Input: part model. Units: mm. Frame: model coordinates. Face numbers are marked on the shaded views. Coordinates: 2 decimals unless noted, no trailing zeros. Loops run counter-clockwise (first coordinate to the right, second up) from the corner with the lowest first, then second, coordinate; pieces in that order, holes last. Notation, with made-up numbers: (56, -23) -> (93, -23) arc R5 cw to (93, -17) -> close; hole circle Ø2 at (-31.75, 76.5). An arc over 180 degrees is marked (long way). Put each result on its own line as item: value. Start each with the question number.
1) Contact query for flat-ended pins moving along their axis: P1, Ø1.8, axis at x = -17.5, z = 3.5, coming from the -Y side; P2, Ø4, axis at x = 48.05, y = 110.5, coming from the -Z side; P3, Ø1.8, axis at y = 118, z = 4.5, coming from the -X side; P4, Ø3, axis at y = 100, z = 2.5, coming from the +X side. Output: stop coordinate, or through.
2) Pull-direction query (X, two-part tool) for the marked faces 1 and 2; classes: pulls with the +X half, pulls with the -X half, needs draft (parallel to the pull), parting line crosses it, or undercut.
3) Cut plane A-A (x = 10.5). Return the cut outline in (y, z), plus the area to 3 significant figures.
4) Cut plane C-C (y = 120.5). Return the cut outline in (x, z), plus the area to 4 significant figures.
5) Cut plane B-B (y = 37). Return the cut outline in (x, z), plus the area to 3 significant figures.
6) Material intervals for L1, parallel to X at y = 150, z = 8.15; L2, parallel to Y at x = -22, z = 4.75; L3, parallel to Y at x = 1.5, z = 7, sorted ascending.
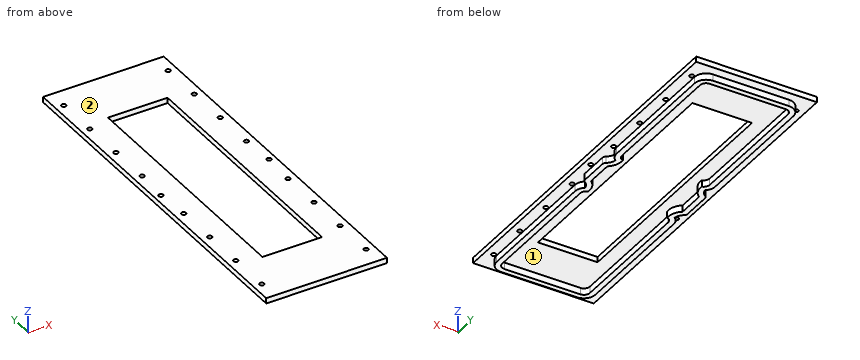
from build123d import *

# Parameters (mm, degrees)
BOSS_EXTRUDE1_DEPTH = 6
BOSS_EXTRUDE2_START = 6
SKETCH1_W           = 111.3
SKETCH1_H           = 338
SKETCH1_R           = 2.1
SKETCH1_W_2         = 54.9
SKETCH1_H_2         = 234
BOSS_EXTRUDE2_DEPTH = 5


with BuildPart() as part:
    # Sketch2 → Boss-Extrude1 (new body)
    with BuildSketch(Plane.XY.offset(0.1)):
        with BuildLine():
            ThreePointArc((-47.25, -13.21070024), (-46.819703068, -14.892045855), (-45.634615385, -16.159975549))
            ThreePointArc((-45.634615385, -16.159975549), (-42.679763233, -19.15303821), (-41.306728934, -23.128507005))
            ThreePointArc((-41.306728934, -23.128507005), (-44.357328362, -26.821736965), (-45.45, -31.485659466))
            Line((-45.45, -31.485659466), (-45.45, -150))
            ThreePointArc((-45.45, -150), (-42.374621202, -157.424621202), (-34.95, -160.5))
            Line((-34.95, -160.5), (34.95, -160.5))
            ThreePointArc((34.95, -160.5), (42.374621202, -157.424621202), (45.45, -150))
            Line((45.45, -150), (45.45, -31.485659466))
            ThreePointArc((45.45, -31.485659466), (44.357328362, -26.821736965), (41.306728934, -23.128507005))
            ThreePointArc((41.306728934, -23.128507005), (42.679763233, -19.15303821), (45.634615385, -16.159975549))
            ThreePointArc((45.634615385, -16.159975549), (46.819703068, -14.892045855), (47.25, -13.21070024))
            Line((47.25, -13.21070024), (47.25, 13.21070024))
            ThreePointArc((47.25, 13.21070024), (46.819703068, 14.892045855), (45.634615385, 16.159975549))
            ThreePointArc((45.634615385, 16.159975549), (42.679763233, 19.15303821), (41.306728934, 23.128507005))
            ThreePointArc((41.306728934, 23.128507005), (44.357328362, 26.821736965), (45.45, 31.485659466))
            Line((45.45, 31.485659466), (45.45, 150))
            ThreePointArc((45.45, 150), (42.374621202, 157.424621202), (34.95, 160.5))
            Line((34.95, 160.5), (-34.95, 160.5))
            ThreePointArc((-34.95, 160.5), (-42.374621202, 157.424621202), (-45.45, 150))
            Line((-45.45, 150), (-45.45, 31.485659466))
            ThreePointArc((-45.45, 31.485659466), (-44.357328362, 26.821736965), (-41.306728934, 23.128507005))
            ThreePointArc((-41.306728934, 23.128507005), (-42.679763233, 19.15303821), (-45.634615385, 16.159975549))
            ThreePointArc((-45.634615385, 16.159975549), (-46.819703068, 14.892045855), (-47.25, 13.21070024))
            Line((-47.25, 13.21070024), (-47.25, -13.21070024))
        make_face()
        with BuildLine():
            ThreePointArc((-40.45, 31.485659466), (-39.318743113, 28.144389705), (-36.390333232, 26.177605191))
            ThreePointArc((-36.390333232, 26.177605191), (-37.409307611, 18.483960794), (-42.25, 12.417811265))
            Line((-42.25, 12.417811265), (-42.25, -12.417811265))
            ThreePointArc((-42.25, -12.417811265), (-37.409307611, -18.483960794), (-36.390333232, -26.177605191))
            ThreePointArc((-36.390333232, -26.177605191), (-39.318743113, -28.144389705), (-40.45, -31.485659466))
            Line((-40.45, -31.485659466), (-40.45, -150))
            ThreePointArc((-40.45, -150), (-38.839087297, -153.889087297), (-34.95, -155.5))
            Line((-34.95, -155.5), (34.95, -155.5))
            ThreePointArc((34.95, -155.5), (38.839087297, -153.889087297), (40.45, -150))
            Line((40.45, -150), (40.45, -31.485659466))
            ThreePointArc((40.45, -31.485659466), (39.318743113, -28.144389705), (36.390333232, -26.177605191))
            ThreePointArc((36.390333232, -26.177605191), (37.409307611, -18.483960794), (42.25, -12.417811265))
            Line((42.25, -12.417811265), (42.25, 12.417811265))
            ThreePointArc((42.25, 12.417811265), (37.409307611, 18.483960794), (36.390333232, 26.177605191))
            ThreePointArc((36.390333232, 26.177605191), (39.318743113, 28.144389705), (40.45, 31.485659466))
            Line((40.45, 31.485659466), (40.45, 150))
            ThreePointArc((40.45, 150), (38.839087297, 153.889087297), (34.95, 155.5))
            Line((34.95, 155.5), (-34.95, 155.5))
            ThreePointArc((-34.95, 155.5), (-38.839087297, 153.889087297), (-40.45, 150))
            Line((-40.45, 150), (-40.45, 31.485659466))
        make_face(mode=Mode.SUBTRACT)
    extrude(amount=BOSS_EXTRUDE1_DEPTH)

    # Sketch1 → Boss-Extrude2 (add)
    with BuildSketch(Plane.XY.offset(0.1).offset(BOSS_EXTRUDE2_START)):
        Rectangle(SKETCH1_W, SKETCH1_H)
        with Locations(Location((49.85, 0, 0), (0, 0, 180))):
            Circle(SKETCH1_R, mode=Mode.SUBTRACT)
        with Locations(Location((48.05, -70.990439644, 0), (0, 0, 180))):
            Circle(SKETCH1_R, mode=Mode.SUBTRACT)
        with Locations(Location((48.05, -110.495219822, 0), (0, 0, 180))):
            Circle(SKETCH1_R, mode=Mode.SUBTRACT)
        with Locations(Location((48.05, -150, 0), (0, 0, 180))):
            Circle(SKETCH1_R, mode=Mode.SUBTRACT)
        with Locations(Location((-48.05, -150, 0), (0, 0, 180))):
            Circle(SKETCH1_R, mode=Mode.SUBTRACT)
        with Locations(Location((-48.05, -110.495219822, 0), (0, 0, 180))):
            Circle(SKETCH1_R, mode=Mode.SUBTRACT)
        with Locations(Location((-48.05, -70.990439644, 0), (0, 0, 180))):
            Circle(SKETCH1_R, mode=Mode.SUBTRACT)
        with Locations(Location((-48.05, 150, 0), (0, 0, 180))):
            Circle(SKETCH1_R, mode=Mode.SUBTRACT)
        with Locations(Location((48.05, 150, 0), (0, 0, 180))):
            Circle(SKETCH1_R, mode=Mode.SUBTRACT)
        with Locations(Location((48.05, 110.495219822, 0), (0, 0, 180))):
            Circle(SKETCH1_R, mode=Mode.SUBTRACT)
        with Locations(Location((-48.05, 110.495219822, 0), (0, 0, 180))):
            Circle(SKETCH1_R, mode=Mode.SUBTRACT)
        with Locations(Location((-48.05, 70.990439644, 0), (0, 0, 180))):
            Circle(SKETCH1_R, mode=Mode.SUBTRACT)
        with Locations(Location((-48.05, 31.485659466, 0), (0, 0, 180))):
            Circle(SKETCH1_R, mode=Mode.SUBTRACT)
        with Locations(Location((48.05, 70.990439644, 0), (0, 0, 180))):
            Circle(SKETCH1_R, mode=Mode.SUBTRACT)
        with Locations(Location((48.05, 31.485659466, 0), (0, 0, 180))):
            Circle(SKETCH1_R, mode=Mode.SUBTRACT)
        with Locations(Location((-49.85, 0, 0), (0, 0, 180))):
            Circle(SKETCH1_R, mode=Mode.SUBTRACT)
        with Locations(Location((-48.05, -31.485659466, 0), (0, 0, 180))):
            Circle(SKETCH1_R, mode=Mode.SUBTRACT)
        with Locations(Location((48.05, -31.485659466, 0), (0, 0, 180))):
            Circle(SKETCH1_R, mode=Mode.SUBTRACT)
        Rectangle(SKETCH1_W_2, SKETCH1_H_2, mode=Mode.SUBTRACT)
    extrude(amount=BOSS_EXTRUDE2_DEPTH)


solid = part.part
Results found:
1. P1: stops at y = -160.5
1. P2: passes through
1. P3: stops at x = -45.45
1. P4: stops at x = 45.45
2. face 1: undercut
2. face 2: needs draft
3. outline: (-169, 6.1) -> (-160.5, 6.1) -> (-160.5, 0.1) -> (-155.5, 0.1) -> (-155.5, 6.1) -> (-117, 6.1) -> (-117, 11.1) -> (-169, 11.1) -> close; (117, 6.1) -> (155.5, 6.1) -> (155.5, 0.1) -> (160.5, 0.1) -> (160.5, 6.1) -> (169, 6.1) -> (169, 11.1) -> (117, 11.1) -> close
3. area: 580 mm2
4. outline: (-55.65, 6.1) -> (-45.45, 6.1) -> (-45.45, 0.1) -> (-40.45, 0.1) -> (-40.45, 6.1) -> (40.45, 6.1) -> (40.45, 0.1) -> (45.45, 0.1) -> (45.45, 6.1) -> (55.65, 6.1) -> (55.65, 11.1) -> (-55.65, 11.1) -> close
4. area: 616.5 mm2
5. outline: (-55.65, 6.1) -> (-45.45, 6.1) -> (-45.45, 0.1) -> (-40.45, 0.1) -> (-40.45, 6.1) -> (-27.45, 6.1) -> (-27.45, 11.1) -> (-55.65, 11.1) -> close; (27.45, 6.1) -> (40.45, 6.1) -> (40.45, 0.1) -> (45.45, 0.1) -> (45.45, 6.1) -> (55.65, 6.1) -> (55.65, 11.1) -> (27.45, 11.1) -> close
5. area: 342 mm2
6. L1: x = -55.65 to -50.15, -45.95 to 45.95, 50.15 to 55.65
6. L2: y = -160.5 to -155.5, 155.5 to 160.5
6. L3: y = -169 to -117, 117 to 169
